Read the model definition and answer for the solid it produces. Units are mm, in the model's axes. A direction names the side the tool comes from. Coordinates: 2 decimals unless noted, no trailing zeros. Write each loop counter-clockwise with the first axis right and the second up, starting at its lowest first coordinate (ties: lowest second). Pieces come first, ordered by that corner, then holes. Notation, with made-up numbers: (46, -27.5) -> (60, -27.5) arc R15 ccw to (60, -10.5) -> close; hole circle Ø11 at (32.5, 55). An arc over 180 degrees is marked (long way). One line per item, written item: value. Start each with the question number.
1. Find section B-B, the plane y = 140.1. Write down the section's boundary in (x, z).
2. Consider line 1 along X through (y, z) = (140.1, 5.5); line 2 along Y through (x, z) = (20, 1.5); line 3 along X through (y, z) = (140.1, 1.3). Determine where each line is inside the solid, lowest interval first.
3. For faces 4 (the flat face through (2, 61, 4)), 5 (the cylindrical face through (16.9, 10.05, 1.01)), 6 (the cylindrical face through (31.15, 137.88, 5.52)), determine the directions among +Z, -Z, +X, -X, +Y, -Y from which every point of the face is accessible in a straight line to the end or side of a thin tool.
4. Given P1, Ø2, axis at x = 30, y = 140.1, coming from the +Z side; P2, Ø11, axis at x = 11, y = 87, coming from the +Z side; P3, Ø6, axis at x = 36, y = 121, coming from the -Z side, each flat-ended and moving along its own axis, determine where each tip first touches the part or whether it passes through.
5. Find section A-A, the plane y = 79. Write down the section's boundary in (x, z), and give its area (3 significant figures).
6. Find section C-C, the plane x = 20. State how many separate pieces and enclosed holes the cut face has, and give its area (3 significant figures).
7. Find section D-D, the plane z = 5.5. Write down the section's boundary in (x, y), and give its area (3 significant figures).
8. For a pull along Y with two mould halves and no side action, classify faces 1 (the cylindrical face through (11.15, 137.88, 5.52)), 2 (the flat face through (20, 61, 2)), 3 (the flat face through (20, 120, 4)) as pulls with the +Y half, pulls with the -Y half, needs draft (parallel to the pull), parting line crosses it, or undercut.
```python
from build123d import *

# Parameters (mm, degrees)
SKETCH1_W           = 40
SKETCH1_H           = 145.1
BOSS_EXTRUDE1_DEPTH = 2
SKETCH2_R           = 14.29
CUT_EXTRUDE1_DEPTH  = 2
BOSS_EXTRUDE2_DEPTH = 5
SKETCH4_R           = 1.25
CUT_EXTRUDE2_DEPTH  = 7
SKETCH5_R           = 2.5
CUT_EXTRUDE3_DEPTH  = 3
SKETCH6_W           = 26
SKETCH6_H           = 12
CUT_EXTRUDE4_DEPTH  = 3


with BuildPart() as part:
    # Sketch1 → Boss-Extrude1 (new body)
    with BuildSketch(Plane.XY):
        with Locations((20, 72.55)):
            Rectangle(SKETCH1_W, SKETCH1_H)
    extrude(amount=BOSS_EXTRUDE1_DEPTH)

    # Sketch2 → Cut-Extrude1 (cut)
    with BuildSketch(Plane.XY.offset(2)):
        with Locations((20, 24)):
            Circle(SKETCH2_R)
    extrude(amount=-CUT_EXTRUDE1_DEPTH, mode=Mode.SUBTRACT)

    # Sketch3 → Boss-Extrude2 (add)
    with BuildSketch(Plane.XY.offset(2)):
        Polygon((0, 145.1), (40, 145.1), (40, 0), (38, 0), (38, 120), (2, 120), (2, 0), (0, 0), align=None)
    extrude(amount=BOSS_EXTRUDE2_DEPTH)

    # Sketch4 → Cut-Extrude2 (cut)
    with BuildSketch(Plane.XY.offset(7)):
        with Locations((20, 140.1)):
            Circle(SKETCH4_R)
        with Locations((10, 140.1)):
            Circle(SKETCH4_R)
        with Locations((30, 140.1)):
            Circle(SKETCH4_R)
    extrude(amount=-CUT_EXTRUDE2_DEPTH, mode=Mode.SUBTRACT)

    # Sketch5 → Cut-Extrude3 (cut)
    with BuildSketch(Plane.XY.offset(7)):
        with Locations((10, 140.1)):
            Circle(SKETCH5_R)
        with Locations((20, 140.1)):
            Circle(SKETCH5_R)
        with Locations((30, 140.1)):
            Circle(SKETCH5_R)
    extrude(amount=-CUT_EXTRUDE3_DEPTH, mode=Mode.SUBTRACT)

    # Sketch6 → Cut-Extrude4 (cut, through all)
    with BuildSketch(Plane.XY.offset(2)):
        with Locations((20, 102)):
            Rectangle(SKETCH6_W, SKETCH6_H)
        with Locations((20, 78)):
            Rectangle(SKETCH6_W, SKETCH6_H)
        with Locations((20, 54)):
            Rectangle(SKETCH6_W, SKETCH6_H)
    extrude(amount=-CUT_EXTRUDE4_DEPTH, mode=Mode.SUBTRACT)


solid = part.part
```
Answer block:
1. outline: (0, 0) -> (8.75, 0) -> (8.75, 4) -> (7.5, 4) -> (7.5, 7) -> (0, 7) -> close; (11.25, 0) -> (18.75, 0) -> (18.75, 4) -> (17.5, 4) -> (17.5, 7) -> (12.5, 7) -> (12.5, 4) -> (11.25, 4) -> close; (21.25, 0) -> (28.75, 0) -> (28.75, 4) -> (27.5, 4) -> (27.5, 7) -> (22.5, 7) -> (22.5, 4) -> (21.25, 4) -> close; (31.25, 0) -> (40, 0) -> (40, 7) -> (32.5, 7) -> (32.5, 4) -> (31.25, 4) -> close
2. line 1: x = 0 to 7.5, 12.5 to 17.5, 22.5 to 27.5, 32.5 to 40
2. line 2: y = 0 to 9.71, 38.29 to 48, 60 to 72, 84 to 96, 108 to 138.85, 141.35 to 145.1
2. line 3: x = 0 to 8.75, 11.25 to 18.75, 21.25 to 28.75, 31.25 to 40
3. face 4: +Z, -Y
3. face 5: +Z, -Z
3. face 6: +Z
4. P1: passes through
4. P2: stops at z = 2
4. P3: stops at z = 0
5. outline: (0, 0) -> (7, 0) -> (7, 2) -> (2, 2) -> (2, 7) -> (0, 7) -> close; (33, 0) -> (40, 0) -> (40, 7) -> (38, 7) -> (38, 2) -> (33, 2) -> close
5. area: 48.0 mm2
6. separate pieces: 6
6. enclosed holes: 0
6. area: 262 mm2
7. outline: (0, 0) -> (2, 0) -> (2, 120) -> (38, 120) -> (38, 0) -> (40, 0) -> (40, 145.1) -> (0, 145.1) -> close; hole circle Ø5 at (10, 140.1); hole circle Ø5 at (20, 140.1); hole circle Ø5 at (30, 140.1)
7. area: 1,430 mm2
8. face 1: undercut
8. face 2: needs draft
8. face 3: pulls with the -Y half
